```python
from build123d import *

# Parameters (mm, degrees)
SKETCH1_W                      = 103
SKETCH1_H                      = 90
BOSS_EXTRUDE1_DEPTH            = 8
FILLET1_R                      = 8
SKETCH7_OUTSIDE_W              = 132.402
SKETCH7_OUTSIDE_H              = 119.402
CUT_EXTRUDE2_DEPTH             = 3
M3X0_5_TAPPED_HOLE1_D          = 2.5
SKETCH15_W                     = 18
SKETCH15_H                     = 50
CUT_EXTRUDE3_DEPTH             = 5
FILLET3_R                      = 2
CBORE_FOR_M4_SHCS1_D           = 4.5
CBORE_FOR_M4_SHCS1_CBORE_D     = 8
CBORE_FOR_M4_SHCS1_CBORE_DEPTH = 4
CBORE_FOR_M3_SHCS2_D           = 3.4
CBORE_FOR_M3_SHCS2_CBORE_D     = 6.5
CBORE_FOR_M3_SHCS2_CBORE_DEPTH = 3
CUT_EXTRUDE4_DEPTH             = 3


with BuildPart() as part:
    # Sketch1 → Boss-Extrude1 (new body)
    with BuildSketch(Plane(origin=(0, 0, 0), x_dir=(1, 0, 0), z_dir=(0, 1, 0))):
        Rectangle(SKETCH1_W, SKETCH1_H)
    extrude(amount=BOSS_EXTRUDE1_DEPTH)

    # Fillet1
    fillet1_edges = [part.edges().sort_by_distance(p)[0] for p in [
        (51.5, 4, 45),
        (-51.5, 4, 45),
        (-51.5, 4, -45),
        (51.5, 4, -45),
    ]]
    fillet(fillet1_edges, radius=FILLET1_R)

    # Sketch7 outside → Cut-Extrude2 (cut)
    with BuildSketch(Plane(origin=(0, 8, 0), x_dir=(1, 0, 0), z_dir=(0, 1, 0))):
        Rectangle(SKETCH7_OUTSIDE_W, SKETCH7_OUTSIDE_H)
        with BuildLine():
            Line((-43.5, -41.6), (43.5, -41.6))
            ThreePointArc((43.5, -41.6), (46.752691193, -40.252691193), (48.1, -37))
            Line((48.1, -37), (48.1, 37))
            ThreePointArc((48.1, 37), (46.752691193, 40.252691193), (43.5, 41.6))
            Line((43.5, 41.6), (-43.5, 41.6))
            ThreePointArc((-43.5, 41.6), (-46.752691193, 40.252691193), (-48.1, 37))
            Line((-48.1, 37), (-48.1, -37))
            ThreePointArc((-48.1, -37), (-46.752691193, -40.252691193), (-43.5, -41.6))
        make_face(mode=Mode.SUBTRACT)
    extrude(amount=-CUT_EXTRUDE2_DEPTH, mode=Mode.SUBTRACT)

    # M3x0.5 Tapped Hole1 (through all)
    with Locations(Plane(origin=(0, 8, 0), x_dir=(1, 0, 0), z_dir=(0, 1, 0))):
        with Locations((-43.5, -37), (-43.5, 37), (43.5, 37), (43.5, -37), (-8.2, 38), (11.2, 38), (30, -1), (10.5, -1)):
            Hole(M3X0_5_TAPPED_HOLE1_D / 2)

    # Sketch15 → Cut-Extrude3 (cut)
    with BuildSketch(Plane(origin=(0, 8, 0), x_dir=(1, 0, 0), z_dir=(0, 1, 0))):
        with Locations((-2.5, -3)):
            Rectangle(SKETCH15_W, SKETCH15_H)
    extrude(amount=-CUT_EXTRUDE3_DEPTH, mode=Mode.SUBTRACT)

    # Fillet3
    fillet3_edges = [part.edges().sort_by_distance(p)[0] for p in [
        (-11.5, 5.5, 28),
        (-11.5, 5.5, -22),
        (6.5, 5.5, -22),
        (6.5, 5.5, 28),
    ]]
    fillet(fillet3_edges, radius=FILLET3_R)

    # CBORE for M4 SHCS1 (through all)
    with Locations(Plane(origin=(0, 0, 0), x_dir=(-1, 0, 0), z_dir=(0, -1, 0))):
        with Locations((17.9, -14), (17.9, 28.5)):
            CounterBoreHole(CBORE_FOR_M4_SHCS1_D / 2, CBORE_FOR_M4_SHCS1_CBORE_D / 2, CBORE_FOR_M4_SHCS1_CBORE_DEPTH)

    # CBORE for M3 SHCS2 (through all)
    with Locations(Plane(origin=(0, 0, 0), x_dir=(-1, 0, 0), z_dir=(0, -1, 0))):
        with Locations((29.087867966, -40.2), (-29, -40.2), (29.087867966, 40.2), (-29, 40.2)):
            CounterBoreHole(CBORE_FOR_M3_SHCS2_D / 2, CBORE_FOR_M3_SHCS2_CBORE_D / 2, CBORE_FOR_M3_SHCS2_CBORE_DEPTH)

    # Sketch21 → Cut-Extrude4 (cut)
    with BuildSketch(Plane(origin=(0, 8, 0), x_dir=(1, 0, 0), z_dir=(0, 1, 0))):
        with BuildLine():
            Line((-30.787867966, 40.2), (-30.787867966, 45))
            ThreePointArc((-30.787867966, 45), (-29.087867966, 46.7), (-27.387867966, 45))
            Line((-27.387867966, 45), (-27.387867966, 40.2))
            ThreePointArc((-27.387867966, 40.2), (-29.087867966, 38.5), (-30.787867966, 40.2))
        make_face()
        with BuildLine():
            Line((27.3, 40.2), (27.3, 45))
            ThreePointArc((27.3, 45), (29, 46.7), (30.7, 45))
            Line((30.7, 45), (30.7, 40.2))
            ThreePointArc((30.7, 40.2), (29, 38.5), (27.3, 40.2))
        make_face()
        with BuildLine():
            Line((-27.387867966, -40.2), (-27.387867966, -45))
            ThreePointArc((-27.387867966, -45), (-29.087867966, -46.7), (-30.787867966, -45))
            Line((-30.787867966, -45), (-30.787867966, -40.2))
            ThreePointArc((-30.787867966, -40.2), (-29.087867966, -38.5), (-27.387867966, -40.2))
        make_face()
        with BuildLine():
            Line((30.7, -40.2), (30.7, -45))
            ThreePointArc((30.7, -45), (29, -46.7), (27.3, -45))
            Line((27.3, -45), (27.3, -40.2))
            ThreePointArc((27.3, -40.2), (29, -38.5), (30.7, -40.2))
        make_face()
    extrude(amount=-CUT_EXTRUDE4_DEPTH, mode=Mode.SUBTRACT)


solid = part.part
```
The model under review builds one solid part; all positions refer to its coordinate system, in mm. A direction names the side the tool comes from. Round coordinates to 2 decimals unless told otherwise and drop trailing zeros. Order: outer loops, then holes, each group sorted by start corner. A loop starts at its lowest first (then second) coordinate and runs counter-clockwise, first axis right, second up.
(1) Mouldability with a two-part tool opening along X and no side actions: class faces 6 (the face through (-20, 4, -27)), 7 (the face through (51.5, 2, 1)), 8 (the face through (37, 7, 41.6)) as released by +X, released by -X, zero draft, split by the parting line, or undercut.
Working result:
face 6: undercut
face 7: released by +X
face 8: zero draft
(2) For P1, Ø2, axis at x = -43.5, z = -37, coming from the -Y side; P2, Ø4, axis at x = 29, z = 40.2, coming from the +Y side; P3, Ø2, axis at x = -28, z = -39, coming from the -Y side; P4, Ø0.9, axis at x = 39, y = 7, coming from the +Z side, all flat-tipped, find the tip position at first contact; note any pin that passes through.
Working result:
P1: passes through
P2: stops at y = 8
P3: stops at y = 3
P4: stops at z = 41.6
(3) Take a section at A-A, the plane y = 1.5. Count the separate pieces of the cut face and the enclosed holes in it, plus the area to 3 significant figures.
Working result:
separate pieces: 1
enclosed holes: 14
area: 8,940 mm2
(4) Wall thickness on L1, parallel to Z at x = 10.5, y = 4; L2, parallel to X at y = 1.65, z = 40.2; L3, parallel to Z at x = 4.5, y = 5.5: over which ranges is each line inside the solid? List them lowest first.
Working result:
L1: z = -45 to -39.04, -36.96 to -0.25, 2.25 to 45
L2: x = -50.83 to -32.34, -25.84 to 25.75, 32.25 to 50.83
L3: z = -41.6 to -22, 28 to 41.6
(5) Take a section at D-D, the plane z = 32.5. State the section outline as (x, y) points, plus the area to 3 significant figures.
Working result:
outline: (-51.5, 0) - (51.5, 0) - (51.5, 5) - (48.1, 5) - (48.1, 8) - (-48.1, 8) - (-48.1, 5) - (-51.5, 5) - close
area: 804 mm2
(6) Take a section at B-B, the plane x = -17.9. State the section outline as (y, z) points, plus the area to 3 significant figures.
Working result:
outline: (0, -45) - (5, -45) - (5, -41.6) - (8, -41.6) - (8, -30.75) - (4, -30.75) - (4, -32.5) - (0, -32.5) - close; (0, -24.5) - (4, -24.5) - (4, -26.25) - (8, -26.25) - (8, 11.75) - (4, 11.75) - (4, 10) - (0, 10) - close; (0, 18) - (4, 18) - (4, 16.25) - (8, 16.25) - (8, 41.6) - (5, 41.6) - (5, 45) - (0, 45) - close
area: 600 mm2
(7) Take a section at C-C, the plane z = 1. State the section outline as (x, y) points.
Working result:
outline: (-51.5, 0) - (9.25, 0) - (9.25, 8) - (6.5, 8) - (6.5, 3) - (-11.5, 3) - (-11.5, 8) - (-48.1, 8) - (-48.1, 5) - (-51.5, 5) - close; (11.75, 0) - (28.75, 0) - (28.75, 8) - (11.75, 8) - close; (31.25, 0) - (51.5, 0) - (51.5, 5) - (48.1, 5) - (48.1, 8) - (31.25, 8) - close
(8) Tool access review of faces 1 (the face through (46.788, 6.521, -40.217)), 2 (the face through (-46.788, 6.521, 40.217)), 3 (the face through (29.423, 1.479, -43.422)), 4 (the face through (-48.1, 7, -1)), 5 (the face through (-3, 6, -22)): name each direction out of +Z, -Z, +X, -X, +Y, -Y from which nothing blocks a thin tool from reaching the whole face with its end or side.
Working result:
face 1: -Z, +X, +Y
face 2: +Z, -X, +Y
face 3: -Y
face 4: +Z, -Z, -X, +Y
face 5: +Y
